Print and shaded views of the part. All mm, measured from the part's lowest x, y and z. Give positions to 0.01 mm unless a question says otherwise; leave off trailing zeros. Write each loop counter-clockwise with the first axis right and the second up, starting at its lowest first coordinate (ties: lowest second). Pieces come first, ordered by that corner, then holes. Notation, with made-up numbers: (14.25, -9.5) -> (40.25, -9.5) arc R23 ccw to (40.25, 28.5) -> close; hole circle Ø6 at (-5, 42.5). An arc over 180 degrees is marked (long way). Put each result on its own line as item: value.
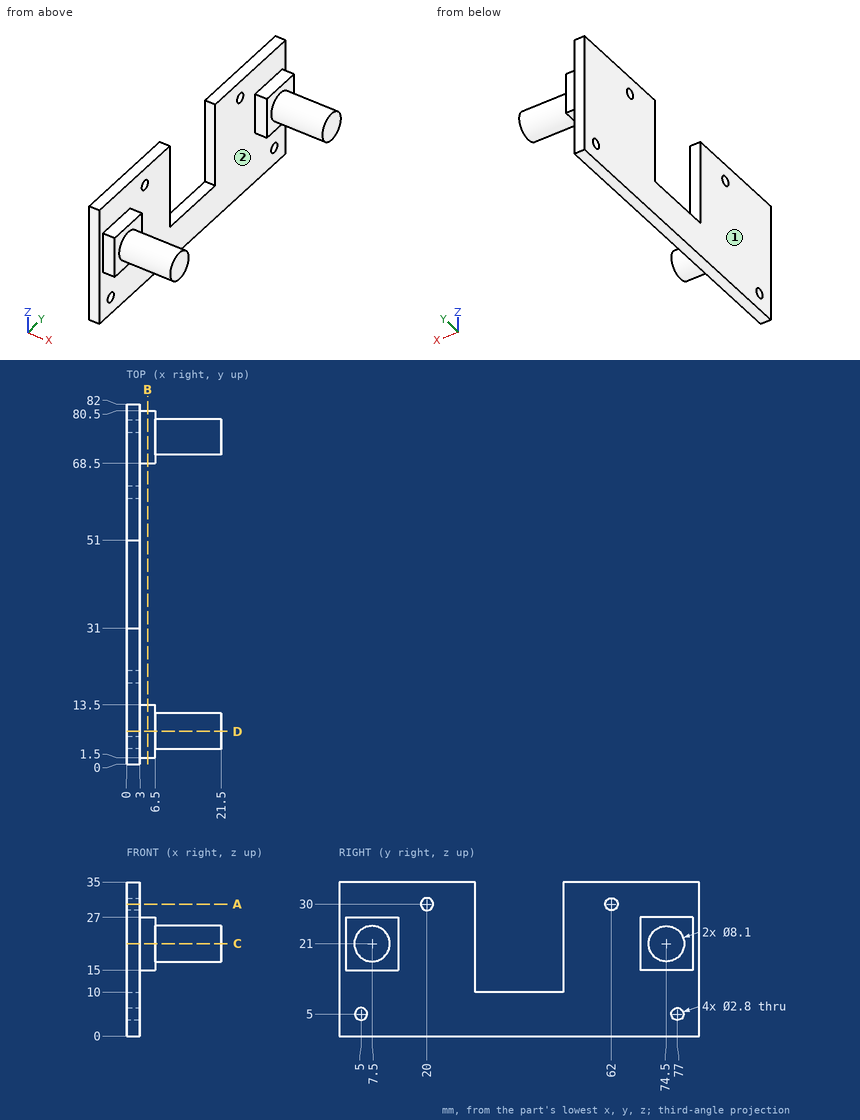
1) Slice it at A-A (z = 30). Write the cut outline in (x, y).
Filled sheet:
outline: (0, 0) -> (3, 0) -> (3, 18.6) -> (0, 18.6) -> close; (0, 21.4) -> (3, 21.4) -> (3, 31) -> (0, 31) -> close; (0, 51) -> (3, 51) -> (3, 60.6) -> (0, 60.6) -> close; (0, 63.4) -> (3, 63.4) -> (3, 82) -> (0, 82) -> close
2) Pin check, flat tips, straight feed: pin 1 (1.8 mm diameter, centred on x = 5, y = 72.5, fed in from -Z); pin 2 (1.5 mm diameter, centred on x = 1.5, z = 16.5, fed in from -Y); pin 3 (6 mm diameter, centred on x = 14.5, z = 16.5, fed in from +Y); pin 4 (6 mm diameter, centred on y = 45.5, z = 4, fed in from +X). Stop position of each tip, or through.
Filled sheet:
pin 1: z = 15
pin 2: y = 0
pin 3: y = 78.26
pin 4: x = 3
3) Pull direction Y, two halves, no side cores. Call the marked faces 1 and 2: released by +Y, released by -Y, zero draft, split by the parting line, or undercut.
Filled sheet:
face 1: zero draft
face 2: undercut
4) Slice it at D-D (y = 7.5). Write the cut outline in (x, z), plus the area to 4 significant figures.
Filled sheet:
outline: (0, 0) -> (3, 0) -> (3, 15) -> (6.5, 15) -> (6.5, 16.95) -> (21.5, 16.95) -> (21.5, 25.05) -> (6.5, 25.05) -> (6.5, 27) -> (3, 27) -> (3, 35) -> (0, 35) -> close
area: 268.5 mm2
5) Slice it at C-C (z = 21). Write the cut outline in (x, y).
Filled sheet:
outline: (0, 0) -> (3, 0) -> (3, 1.5) -> (6.5, 1.5) -> (6.5, 3.45) -> (21.5, 3.45) -> (21.5, 11.55) -> (6.5, 11.55) -> (6.5, 13.5) -> (3, 13.5) -> (3, 31) -> (0, 31) -> close; (0, 51) -> (3, 51) -> (3, 68.5) -> (6.5, 68.5) -> (6.5, 70.45) -> (21.5, 70.45) -> (21.5, 78.55) -> (6.5, 78.55) -> (6.5, 80.5) -> (3, 80.5) -> (3, 82) -> (0, 82) -> close
6) Slice it at B-B (x = 4.75). Write the cut outline in (y, z).
Filled sheet:
outline: (1.5, 15) -> (13.5, 15) -> (13.5, 27) -> (1.5, 27) -> close; (68.5, 15) -> (80.5, 15) -> (80.5, 27) -> (68.5, 27) -> close
7) Wall check: L1, parallel to Y at x = 2.1, z = 30; L2, parallel to Y at x = 2.25, z = 5; L3, parallel to Y at x = 9.5, z = 21. Give the ranges that are in metal, low to high.
Filled sheet:
L1: 0 to 18.6, 21.4 to 31, 51 to 60.6, 63.4 to 82
L2: 0 to 3.6, 6.4 to 75.6, 78.4 to 82
L3: 3.45 to 11.55, 70.45 to 78.55
